Could you check a few things on this model? Use its own coordinates, in mm. A direction names the side the tool comes from. Round coordinates to 2 decimals unless told otherwise and drop trailing zeros. Write each loop counter-clockwise with the first axis right and the second up, starting at its lowest first coordinate (ties: lowest second). Pieces come first, ordered by that corner, then holes. Notation, with made-up numbers: (21, -39.75) -> (74, -39.75) arc R34 cw to (74, -6.75) -> close; hole circle Ø2 at (59.25, 86). An arc over 180 degrees is marked (long way). One line per question, with ' | ' between items. Start each with the question number.
1. For pin 1 Ø4 at (y, z) = (-3, 9) entering from -X; pin 2 Ø5.5 at (x, z) = (13, 13.5) entering from -Y; pin 3 Ø3 at (x, z) = (-4, 9.5) entering from -Y; pin 4 Ø2.5 at (x, y) = (26.37, 5.8) entering from -Z, each with a flat end and sliding along its axis, tell me the tip position at first contact or that it passes through.
2. Imagine slicing it at A-A, the plane z = 1.75. List the corners of the cut face in (x, y) for me, and give its area (3 significant figures).
3. Imagine slicing it at B-B, the plane z = 11.75. State how many separate pieces and enclosed holes the cut face has, and give its area (3 significant figures).
4. Thinking about a two-plate mould opening in Y: for faces 6 (the flat face through (-16.83, 4.04, 11.76)), 7 (the flat face through (30, 2, 8)), 8 (the cylindrical face through (16.05, -7.7, 7.74)), which applies, released by +Y, released by -Y, zero draft, split by the parting line, or undercut?
5. For faces 1 (the flat face through (14, 0.325, 12)), 2 (the cylindrical face through (-28.182, 5.229, 7.74)), 3 (the cylindrical face through (29.264, -2.689, 5.996)), 4 (the flat face through (15, -3, 6)), 5 (the cylindrical face through (-7.607, 5.392, 11.756)), which set-ups out of +Z, -Z, +X, -X, +Y, -Y let a thin tool reach every point of the face, with its end or its side?
6. If I drill on line 1 along X through (y, z) = (5, 4); line 2 along Y through (x, z) = (-19.27, 8); line 3 along X through (y, z) = (-5.2, 9) (3 decimals), over which ranges is the centre line in solid material (lowest first)? Write a range as [from, to].
from build123d import *

# Parameters (mm, degrees)
F1_DEPTH    = 15.7
F2_W        = 10.0960650777
F2_H        = 2.4
F3_DEPTH    = 8
F4_R        = 5
F5_T1_DEPTH = 26.8923143391
F5_T3_DEPTH = 21.3473434867
F5_T5_DEPTH = 35.7
F6_W        = 15
F6_H        = 6.25
F7_DEPTH    = 2
F8_SIZE     = 1.99999


# Not quite as in the source:
# - a fillet or chamfer that OpenCascade refuses, or shapes differently, is made with other operations: its cross-section is extruded or revolved along the edge and cut away or added
# - a fillet or chamfer is up to 0.001 mm smaller than in the source, because OpenCascade refuses the exact size


with BuildPart() as f1:
    # F0 (on Top) → F1 (new body)
    with BuildSketch(Plane.XY):
        Polygon((30, 9), (0, 9), (0, -1.8), (15, -1.8), (15, -9), (19.5954625243, -9), (30, -2.6151265483), align=None)
        with BuildLine():
            ThreePointArc((21.17, -5.2), (17.9264971157, -6.5435028843), (19.27, -3.3))
            ThreePointArc((19.27, -3.3), (20.6135028843, -3.8564971157), (21.17, -5.2))
        make_face(mode=Mode.SUBTRACT)
        with BuildLine():
            ThreePointArc((19.27, 3.9), (17.9264971157, 7.1435028843), (21.17, 5.8))
            ThreePointArc((21.17, 5.8), (20.6135028843, 4.4564971157), (19.27, 3.9))
        make_face(mode=Mode.SUBTRACT)
        with BuildLine():
            ThreePointArc((24.47, 5.8), (26.37, 7.7), (28.27, 5.8))
            ThreePointArc((28.27, 5.8), (26.37, 3.9), (24.47, 5.8))
        make_face(mode=Mode.SUBTRACT)
    extrude(amount=F1_DEPTH)

    # F2 (on face) → F3 (cut)
    with BuildSketch(Plane.XY.offset(15.7)):
        with BuildLine():
            ThreePointArc((11.6039349223, 0.3250306588), (9.2827431951, 3.7535073497), (13.3280728534, 4.6353754864))
            Line((13.3280728534, 4.6353754864), (16.2527744297, 1.8499454137))
            ThreePointArc((16.2527744297, 1.8499454137), (16.328577113, 2.3348713274), (16.3539349223, 2.8250306588))
            ThreePointArc((16.3539349223, 2.8250306588), (16.0563093355, 4.479981439), (15.200729834, 5.9275403467))
            ThreePointArc((15.200729834, 5.9275403467), (7.5407755063, 5.2853630672), (10.5215341623, -1.8))
            Line((10.5215341623, -1.8), (12.6863356823, -1.8))
            ThreePointArc((12.6863356823, -1.8), (14.376262754, -1.0320016711), (15.6428085277, 0.3250306588))
            Line((15.6428085277, 0.3250306588), (11.6039349223, 0.3250306588))
        make_face()
        with BuildLine():
            ThreePointArc((16.3539349223, 2.8250306588), (16.328577113, 2.3348713274), (16.2527744297, 1.8499454137))
            Line((16.2527744297, 1.8499454137), (16.9487625085, 1.1870996243))
            ThreePointArc((16.9487625085, 1.1870996243), (17.0635074373, 1.0219903081), (17.1039349223, 0.8250306588))
            ThreePointArc((17.1039349223, 0.8250306588), (16.9574883129, 0.4714772682), (16.6039349223, 0.3250306588))
            Line((16.6039349223, 0.3250306588), (15.6428085277, 0.3250306588))
            ThreePointArc((15.6428085277, 0.3250306588), (14.376262754, -1.0320016711), (12.6863356823, -1.8))
            Line((12.6863356823, -1.8), (15, -1.8))
            Line((15, -1.8), (15, -1.9249693412))
            Line((15, -1.9249693412), (19.9039349223, -1.9249693412))
            Line((19.9039349223, -1.9249693412), (19.9039349223, 0.4750306588))
            Line((19.9039349223, 0.4750306588), (15.200729834, 5.9275403467))
            ThreePointArc((15.200729834, 5.9275403467), (16.0563093355, 4.479981439), (16.3539349223, 2.8250306588))
        make_face()
        with Locations((24.9519674612, -0.7249693412)):
            Rectangle(F2_W, F2_H)
    extrude(amount=-F3_DEPTH, mode=Mode.SUBTRACT)

    # F4
    f4_edges = [f1.edges().sort_by_distance(p)[0] for p in [
        (19.903935, 0.475031, 11.7),
    ]]
    fillet(f4_edges, radius=F4_R)

    # F5: fillet of radius 4 on 4 edges, made by hand

    # F5_s2 → F5_t1 (cut)
    with BuildSketch(Plane.XY.offset(-5.5961571696)):
        with BuildLine():
            ThreePointArc((30, -0.3766636805), (29.4905957559, -2.3300559271), (28.0921293656, -3.7859150232))
            Line((28.0921293656, -3.7859150232), (30, -2.6151265483))
            Line((30, -2.6151265483), (30, -0.3766636805))
        make_face()
    extrude(amount=F5_T1_DEPTH, mode=Mode.SUBTRACT)

    # F5_s4 → F5_t3 (cut)
    with BuildSketch(Plane.XY.offset(-2.8236717433)):
        with BuildLine():
            ThreePointArc((20.5581231925, -8.4092513427), (19.5529608525, -8.8494808332), (18.465993827, -9))
            Line((18.465993827, -9), (19.5954625243, -9))
            Line((19.5954625243, -9), (20.5581231925, -8.4092513427))
        make_face()
    extrude(amount=F5_T3_DEPTH, mode=Mode.SUBTRACT)

    # F5_s6 → F5_t5 (cut)
    with BuildSketch(Plane.XY.offset(-10)):
        with BuildLine():
            ThreePointArc((15, -5), (16.1715728753, -7.8284271247), (19, -9))
            Line((19, -9), (15, -9))
            Line((15, -9), (15, -5))
        make_face()
        with BuildLine():
            ThreePointArc((30, 5), (28.8284271247, 7.8284271247), (26, 9))
            Line((26, 9), (30, 9))
            Line((30, 9), (30, 5))
        make_face()
    extrude(amount=F5_T5_DEPTH, mode=Mode.SUBTRACT)

    # F6 (on face) → F7 (cut)
    with BuildSketch(Plane.XZ.offset(1.8)):
        with Locations((7.5, 3.125)):
            Rectangle(F6_W, F6_H)
    extrude(amount=-F7_DEPTH, mode=Mode.SUBTRACT)

    # F8 (size 2 in the source; OpenCascade refuses exactly that, so slightly less here)
    f8_edges = [f1.edges().sort_by_distance(p)[0] for p in [
        (7.5, 0.2, 6.25),
    ]]
    chamfer(f8_edges, length=F8_SIZE)

    # F9: F1 across plane


with BuildPart() as f1_1:
    add(f1.part)
    add(f1.part.mirror(Plane.YZ))


solid = f1_1.part
Geometry results:
1) pin 1: stops at x = -29.84 | pin 2: stops at y = -7.33 | pin 3: stops at y = -1.8 | pin 4: passes through
2) outline: (-30, -0.38) arc R4 ccw to (-28.09, -3.79) -> (-20.56, -8.41) arc R4 ccw to (-18.73, -8.99) arc R4 ccw to (-15, -5) -> (-15, 0.2) -> (15, 0.2) -> (15, -5) arc R4 ccw to (18.73, -8.99) arc R4 ccw to (20.56, -8.41) -> (28.09, -3.79) arc R4 ccw to (30, -0.38) -> (30, 5) arc R4 ccw to (26, 9) -> (-26, 9) arc R4 ccw to (-30, 5) -> close; hole circle Ø3.8 at (-26.37, 5.8); hole circle Ø3.8 at (-19.27, -5.2); hole circle Ø3.8 at (-19.27, 5.8); hole circle Ø3.8 at (19.27, -5.2); hole circle Ø3.8 at (19.27, 5.8); hole circle Ø3.8 at (26.37, 5.8) | area: 654 mm2
3) separate pieces: 5 | enclosed holes: 6 | area: 537 mm2
4) face 6: undercut | face 7: zero draft | face 8: released by -Y
5) face 1: +Z, +X | face 2: +Z, -Z | face 3: +Z, -Z, +X, -Y | face 4: -Z, -Y | face 5: +Z
6) line 1: x = [-30, -28.09], [-24.65, -20.99], [-17.55, 17.55], [20.99, 24.65], [28.09, 30] | line 2: y = [-8.92, -7.1], [-3.3, -1.92], [1.42, 3.9], [7.7, 9] | line 3: x = [-25.788, -21.17], [-17.37, -15.005], [15.005, 17.37], [21.17, 25.788]
